Could you check a few things on this model? Use its own coordinates, in mm. Face numbers are marked on the shaded views. Round coordinates to 2 decimals unless told otherwise and drop trailing zeros. Write each loop counter-clockwise with the first axis right and the second up, starting at its lowest first coordinate (ties: lowest second). Pieces come first, ordered by that corner, then holes. Notation, with made-up numbers: M -22.75,16.25 L 23.25,16.25 A10 ccw 23.25,20.25 Z; hole C 62.25,22.25 d10. An arc over 180 degrees is marked long. One line per item, written item: value. Start each with the question number.
(1) I want a section at A-A on y = 0. Please give me the cut outline in (x, z).
(2) Thinking about a two-plate mould opening in Z: for the marked faces 1, 2 and 3, which applies, released by +Z, released by -Z, zero draft, split by the parting line, or undercut?
(3) I want a section at C-C on x = 304. Count the separate pieces of the cut face and the enclosed holes in it, and give its area (3 significant figures).
(4) I'm going to push flat-ended pins straight in: pin 1 Ø8 at (y, z) = (-22.5, 5) entering from -X; pin 2 Ø1 at (x, z) = (326.5, 25.5) entering from -Y; pin 3 Ø2.5 at (y, z) = (30, 50.5) entering from -X; pin 4 Ø2 at (x, y) = (306.5, 20.5) entering from +Z. Where does each tip first touch, or does it pass through?
(5) If I drill on L1, parallel to Z at x = 304.5, y = 0; L2, parallel to Z at x = 294.5, y = 0; L3, parallel to Y at x = 339.5, z = 10.5, over which ranges is the centre line in solid material (lowest first)?
(6) I want a section at D-D on z = 59.69. Please give me the cut outline in (x, y).
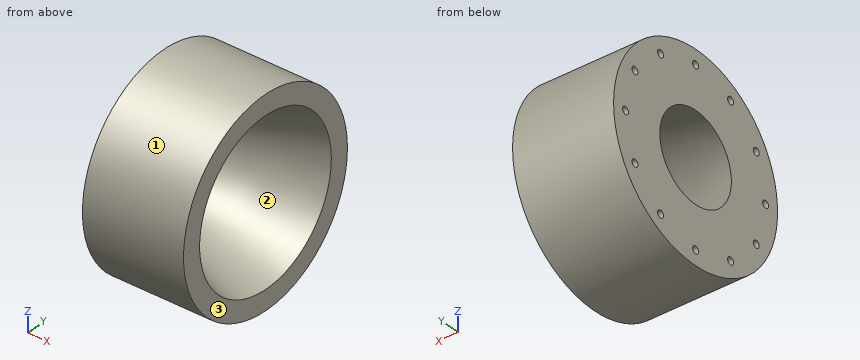
```python
from build123d import *

# Parameters (mm, degrees)
SKETCH4_R          = 2.54
CUT_EXTRUDE1_DEPTH = 30.48
CIRPATTERN1_COUNT  = 12


with BuildPart() as part:
    # Sketch1 → Revolve1 (revolve)
    with BuildSketch(Plane.XY):
        Polygon((280.911030354, 30.48), (351.369552102, 56.124804667), (351.369552102, 69.85), (280.911030354, 69.85), (280.911030354, 50.8), align=None)
    revolve(axis=Axis((0, 0, 0), (1, 0, 0)))

    # Sketch4 → Cut-Extrude1 (cut)
    with BuildSketch(Plane.ZY.offset(-280.911030354)):
        with Locations((0, 59.69)):
            Circle(SKETCH4_R)
    cut_extrude1 = extrude(amount=-CUT_EXTRUDE1_DEPTH, mode=Mode.SUBTRACT)

    # CirPattern1: Cut-Extrude1 ×12 about axis
    cirpattern1_axis = Axis((0, 0, 0), (1, 0, 0))
    for i in range(1, CIRPATTERN1_COUNT):
        add(cut_extrude1.rotate(cirpattern1_axis, i * 360 / CIRPATTERN1_COUNT), mode=Mode.SUBTRACT)


solid = part.part
```
Found:
1. outline: M 280.91,-69.85 L 351.37,-69.85 L 351.37,-56.12 L 280.91,-30.48 L 280.91,-57.15 L 311.39,-57.15 L 311.39,-62.23 L 280.91,-62.23 Z; M 280.91,30.48 L 351.37,56.12 L 351.37,69.85 L 280.91,69.85 L 280.91,62.23 L 311.39,62.23 L 311.39,57.15 L 280.91,57.15 Z
2. face 1: split by the parting line
2. face 2: undercut
2. face 3: zero draft
3. separate pieces: 1
3. enclosed holes: 13
3. area: 10,300 mm²
4. pin 1: passes through
4. pin 2: stops at y = -65.22
4. pin 3: stops at x = 311.39
4. pin 4: stops at z = 67.07
5. L1: z = -69.85 to -62.23, -57.15 to -39.07, 39.07 to 57.15, 62.23 to 69.85
5. L2: z = -69.85 to -62.23, -57.15 to -35.43, 35.43 to 57.15, 62.23 to 69.85
5. L3: y = -69.06 to -50.73, 50.73 to 69.06
6. outline: M 280.91,-36.28 L 351.37,-36.28 L 351.37,36.28 L 280.91,36.28 L 280.91,2.54 L 311.39,2.54 L 311.39,-2.54 L 280.91,-2.54 Z
